Verification items for the finished model (mm, model axes). Round coordinates to 2 decimals unless told otherwise and drop trailing zeros. Order: outer loops, then holes, each group sorted by start corner. A loop starts at its lowest first (then second) coordinate and runs counter-clockwise, first axis right, second up. Notation, with made-up numbers: M -35.75,-35.5 L -25.75,-35.5 A18 cw -25.75,-7.5 Z; hole C 64.5,58.5 d7. An arc over 180 degrees is marked long. Use CSV: the item, a comma, the result in double quotes. Start each with the question number.
Q1. Sectioned sample at C-C (x = -2.75). Enter the section's corners in (y, z).
Q2. Sectioned sample at B-B (y = 4.7). Enter the section's corners in (x, z), and give its area (3 significant figures).
Q3. Sectioned sample at A-A (x = 0). Enter the section's corners in (y, z), and give its area (3 significant figures).
Q4. Scan lines: line 1 (Y direction, x = 0, z = -0.15); line 2 (X direction, y = 1.25, z = 0.45); line 3 (X direction, y = -4.5, z = -0.3). Record each from-to range of solid material in increasing order.
Q5. Gauge pin test, flat ends, axial feed: pin 1 Ø1.8 at (x, y) = (0, -4.7) entering from +Z; pin 2 Ø4 at (x, y) = (0, 0) entering from -Z. Record the tip position at first contact, or that the pin passes through.
Q6. Sectioned sample at D-D (x = -6.5). Enter the section's corners in (y, z).
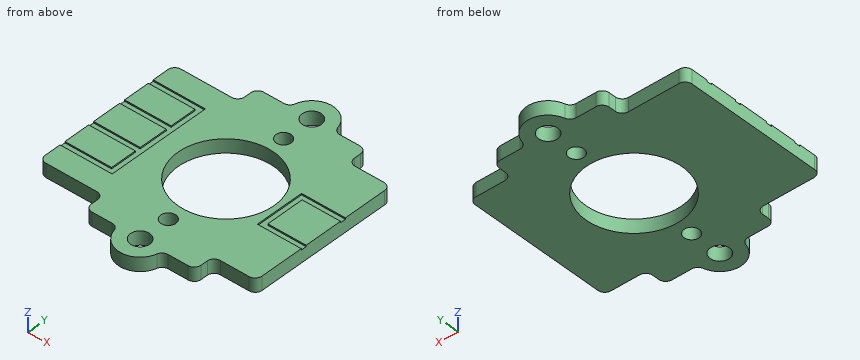
```python
from build123d import *

# Parameters (mm, degrees)
MODEL_R         = 3.5
MODEL_R_2       = 0.7
EXTRUDE_1_DEPTH = 0.5
EXTRUDE2_DEPTH  = 0.1
SKETCH3_R       = 0.55
EXTRUDE3_DEPTH  = 13.273956167


with BuildPart() as part:
    # Model → Бобышка-Вытянуть1 (new, symmetric)
    with BuildSketch(Plane.XY):
        with BuildLine():
            Line((-3.5, 7), (-2.039607805, 7))
            ThreePointArc((-2.039607805, 7), (-1.731001106, 7.106602104), (-1.553986899, 7.380952381))
            ThreePointArc((-1.553986899, 7.380952381), (0, 8.6), (1.553986899, 7.380952381))
            ThreePointArc((1.553986899, 7.380952381), (1.731001106, 7.106602104), (2.039607805, 7))
            Line((2.039607805, 7), (3.5, 7))
            ThreePointArc((3.5, 7), (3.853553391, 6.853553391), (4, 6.5))
            Line((4, 6.5), (4, 6))
            ThreePointArc((4, 6), (4.146446609, 5.646446609), (4.5, 5.5))
            Line((4.5, 5.5), (6.6, 5.5))
            ThreePointArc((6.6, 5.5), (6.953553391, 5.353553391), (7.1, 5))
            Line((7.1, 5), (7.1, -5))
            ThreePointArc((7.1, -5), (6.953553391, -5.353553391), (6.6, -5.5))
            Line((6.6, -5.5), (4.5, -5.5))
            ThreePointArc((4.5, -5.5), (4.146446609, -5.646446609), (4, -6))
            Line((4, -6), (4, -6.5))
            ThreePointArc((4, -6.5), (3.853553391, -6.853553391), (3.5, -7))
            Line((3.5, -7), (2.039607805, -7))
            ThreePointArc((2.039607805, -7), (1.731001106, -7.106602104), (1.553986899, -7.380952381))
            ThreePointArc((1.553986899, -7.380952381), (0, -8.6), (-1.553986899, -7.380952381))
            ThreePointArc((-1.553986899, -7.380952381), (-1.731001106, -7.106602104), (-2.039607805, -7))
            Line((-2.039607805, -7), (-3.5, -7))
            ThreePointArc((-3.5, -7), (-3.853553391, -6.853553391), (-4, -6.5))
            Line((-4, -6.5), (-4, -6))
            ThreePointArc((-4, -6), (-4.146446609, -5.646446609), (-4.5, -5.5))
            Line((-4.5, -5.5), (-8.2, -5.5))
            ThreePointArc((-8.2, -5.5), (-8.553553391, -5.353553391), (-8.7, -5))
            Line((-8.7, -5), (-8.7, 5))
            ThreePointArc((-8.7, 5), (-8.553553391, 5.353553391), (-8.2, 5.5))
            Line((-8.2, 5.5), (-4.5, 5.5))
            ThreePointArc((-4.5, 5.5), (-4.146446609, 5.646446609), (-4, 6))
            Line((-4, 6), (-4, 6.5))
            ThreePointArc((-4, 6.5), (-3.853553391, 6.853553391), (-3.5, 7))
        make_face()
        Circle(MODEL_R, mode=Mode.SUBTRACT)
        with Locations((0, 7)):
            Circle(MODEL_R_2, mode=Mode.SUBTRACT)
        with Locations((0, -7)):
            Circle(MODEL_R_2, mode=Mode.SUBTRACT)
    extrude(amount=EXTRUDE_1_DEPTH, both=True)

    # Sketch2 → Extrude2 (cut)
    with BuildSketch(Plane.XY.offset(0.5)):
        Polygon((-9.557418436, -3.8), (-4.9, -3.8), (-4.9, 3.8), (-9.557418436, 3.8), (-9.557418436, 3.4), (-5.3, 3.4), (-5.3, 1.462476295), (-9.557418436, 1.462476295), (-9.557418436, 1.062476295), (-5.3, 1.062476295), (-5.3, -1.062476295), (-9.557418436, -1.062476295), (-9.557418436, -1.462476295), (-5.3, -1.462476295), (-5.3, -3.4), (-9.557418436, -3.4), align=None)
        Polygon((7.739654587, -1.8), (7.739654587, -1.4), (4.3, -1.4), (4.3, 1.4), (7.739654587, 1.4), (7.739654587, 1.8), (3.9, 1.8), (3.9, -1.8), align=None)
    extrude(amount=-EXTRUDE2_DEPTH, mode=Mode.SUBTRACT)

    # Sketch3 → Extrude3 (cut, through all)
    with BuildSketch(Plane.XY.offset(0.5)):
        with Locations((0, 4.7)):
            Circle(SKETCH3_R)
        with Locations((0, -4.7)):
            Circle(SKETCH3_R)
    extrude(amount=-EXTRUDE3_DEPTH, mode=Mode.SUBTRACT)


solid = part.part
```
Verdict:
1,outline,"M -7,-0.5 L -2.17,-0.5 L -2.17,0.5 L -7,0.5 Z; M 2.17,-0.5 L 7,-0.5 L 7,0.5 L 2.17,0.5 Z"
2,outline,"M -8.7,-0.5 L -0.55,-0.5 L -0.55,0.5 L -8.7,0.5 Z; M 0.55,-0.5 L 7.1,-0.5 L 7.1,0.5 L 0.55,0.5 Z"
2,area,"14.7 mm²"
3,outline,"M -8.6,-0.5 L -7.7,-0.5 L -7.7,0.5 L -8.6,0.5 Z; M -6.3,-0.5 L -5.25,-0.5 L -5.25,0.5 L -6.3,0.5 Z; M -4.15,-0.5 L -3.5,-0.5 L -3.5,0.5 L -4.15,0.5 Z; M 3.5,-0.5 L 4.15,-0.5 L 4.15,0.5 L 3.5,0.5 Z; M 5.25,-0.5 L 6.3,-0.5 L 6.3,0.5 L 5.25,0.5 Z; M 7.7,-0.5 L 8.6,-0.5 L 8.6,0.5 L 7.7,0.5 Z"
3,area,"5.20 mm²"
4,line 1,"y = -8.6 to -7.7, -6.3 to -5.25, -4.15 to -3.5, 3.5 to 4.15, 5.25 to 6.3, 7.7 to 8.6"
4,line 2,"x = -4.9 to -3.27, 3.27 to 3.9, 4.3 to 7.1"
4,line 3,"x = -8.7 to -0.51, 0.51 to 7.1"
5,pin 1,"stops at z = 0.5"
5,pin 2,"passes through"
6,outline,"M -5.5,-0.5 L 5.5,-0.5 L 5.5,0.5 L 3.8,0.5 L 3.8,0.4 L 3.4,0.4 L 3.4,0.5 L 1.46,0.5 L 1.46,0.4 L 1.06,0.4 L 1.06,0.5 L -1.06,0.5 L -1.06,0.4 L -1.46,0.4 L -1.46,0.5 L -3.4,0.5 L -3.4,0.4 L -3.8,0.4 L -3.8,0.5 L -5.5,0.5 Z"
